```python
from build123d import *

# Parameters (mm, degrees)
CORTAR_EXTRUIR2_DEPTH = 112
CROQUIS11_W           = 4
CROQUIS11_H           = 16.808089165
CROQUIS11_W_2         = 16.808089165
CROQUIS11_H_2         = 4
CORTAR_EXTRUIR3_DEPTH = 40


with BuildPart() as part:
    # Croquis1 → Revolución1 (revolve)
    with BuildSketch(Plane.XY):
        Polygon((-27.489415048, 0), (-30, 0), (-30, -1), (-28.5, -1), (-27.603353842, -11), (-26.603353842, -11), (-22, -60), (0, -60), (0, -58.902540381), (-21.020029368, -58.902540381), (-25.804439037, -9.881949504), (-26.603353842, -9.881949504), align=None)
    revolve(axis=Axis((0, -60, 0), (0, 1, 0)))

    # Croquis9 → Cortar-Extruir2 (cut)
    with BuildSketch(Plane(origin=(0, 0, 0), x_dir=(1, 0, 0), z_dir=(0, 1, 0))):
        with BuildLine():
            Line((-1.75, 6.184718181), (-1.5, 19.300075922))
            ThreePointArc((-1.5, 19.300075922), (-7.408092304, 17.884716912), (-12.58655439, 14.707874734))
            Line((-12.58655439, 14.707874734), (-3.135819299, 5.610693033))
            ThreePointArc((-3.135819299, 5.610693033), (-2.459712132, 5.938270389), (-1.75, 6.184718181))
        make_face()
        with BuildLine():
            Line((3.135819299, 5.610693033), (12.58655439, 14.707874734))
            ThreePointArc((12.58655439, 14.707874734), (7.408092304, 17.884716912), (1.5, 19.300075922))
            Line((1.5, 19.300075922), (1.75, 6.184718181))
            ThreePointArc((1.75, 6.184718181), (2.459712132, 5.938270389), (3.135819299, 5.610693033))
        make_face()
        with BuildLine():
            Line((6.184718181, 1.75), (19.300075922, 1.5))
            ThreePointArc((19.300075922, 1.5), (17.884716912, 7.408092304), (14.707874734, 12.58655439))
            Line((14.707874734, 12.58655439), (5.610693033, 3.135819299))
            ThreePointArc((5.610693033, 3.135819299), (5.938270389, 2.459712132), (6.184718181, 1.75))
        make_face()
        with BuildLine():
            Line((5.610693033, -3.135819299), (14.707874734, -12.58655439))
            ThreePointArc((14.707874734, -12.58655439), (17.884716912, -7.408092304), (19.300075922, -1.5))
            Line((19.300075922, -1.5), (6.184718181, -1.75))
            ThreePointArc((6.184718181, -1.75), (5.938270389, -2.459712132), (5.610693033, -3.135819299))
        make_face()
        with BuildLine():
            Line((1.75, -6.184718181), (1.5, -19.300075922))
            ThreePointArc((1.5, -19.300075922), (7.408092304, -17.884716912), (12.58655439, -14.707874734))
            Line((12.58655439, -14.707874734), (3.135819299, -5.610693033))
            ThreePointArc((3.135819299, -5.610693033), (2.459712132, -5.938270389), (1.75, -6.184718181))
        make_face()
        with BuildLine():
            Line((-3.135819299, -5.610693033), (-12.58655439, -14.707874734))
            ThreePointArc((-12.58655439, -14.707874734), (-7.408092304, -17.884716912), (-1.5, -19.300075922))
            Line((-1.5, -19.300075922), (-1.75, -6.184718181))
            ThreePointArc((-1.75, -6.184718181), (-2.459712132, -5.938270389), (-3.135819299, -5.610693033))
        make_face()
        with BuildLine():
            Line((-6.184718181, -1.75), (-19.300075922, -1.5))
            ThreePointArc((-19.300075922, -1.5), (-17.884716912, -7.408092304), (-14.707874734, -12.58655439))
            Line((-14.707874734, -12.58655439), (-5.610693033, -3.135819299))
            ThreePointArc((-5.610693033, -3.135819299), (-5.938270389, -2.459712132), (-6.184718181, -1.75))
        make_face()
        with BuildLine():
            Line((-5.610693033, 3.135819299), (-14.707874734, 12.58655439))
            ThreePointArc((-14.707874734, 12.58655439), (-17.884716912, 7.408092304), (-19.300075922, 1.5))
            Line((-19.300075922, 1.5), (-6.184718181, 1.75))
            ThreePointArc((-6.184718181, 1.75), (-5.938270389, 2.459712132), (-5.610693033, 3.135819299))
        make_face()
    extrude(amount=-CORTAR_EXTRUIR2_DEPTH, mode=Mode.SUBTRACT)

    # Croquis11 → Cortar-Extruir3 (cut)
    with BuildSketch(Plane(origin=(0, -56, 0), x_dir=(1, 0, 0), z_dir=(0, 1, 0))):
        with Locations((-0.4, 22.457977408)):
            Rectangle(CROQUIS11_W, CROQUIS11_H)
        Polygon((9.372703114, 29.283983817), (2.940525861, 13.755334257), (6.636043991, 12.224600528), (13.068221244, 27.753250088), align=None)
        Polygon((19.645373498, 23.320848212), (7.760259671, 11.435734384), (10.588686796, 8.60730726), (22.473800623, 20.492421087), align=None)
        Polygon((26.854090209, 13.880448514), (11.325440649, 7.448271261), (12.856174379, 3.75275313), (28.384823939, 10.184930384), align=None)
        with Locations((21.497346893, 0.4)):
            Rectangle(CROQUIS11_W_2, CROQUIS11_H_2)
        Polygon((28.323353302, -9.372703114), (12.794703741, -2.940525861), (11.263970012, -6.636043991), (26.792619572, -13.068221244), align=None)
        Polygon((22.360217696, -19.645373498), (10.475103869, -7.760259671), (7.646676744, -10.588686796), (19.531790571, -22.473800623), align=None)
        Polygon((12.919817998, -26.854090209), (6.487640745, -11.325440649), (2.792122615, -12.856174379), (9.224299868, -28.384823939), align=None)
        with Locations((-0.560630516, -21.497346893)):
            Rectangle(CROQUIS11_W, CROQUIS11_H)
        Polygon((-10.333333629, -28.323353302), (-3.901156376, -12.794703741), (-7.596674506, -11.263970012), (-14.028851759, -26.792619572), align=None)
        Polygon((-20.606004014, -22.360217696), (-8.720890187, -10.475103869), (-11.549317311, -7.646676744), (-23.434431139, -19.531790571), align=None)
        Polygon((-27.814720725, -12.919817998), (-12.286071165, -6.487640745), (-13.816804894, -2.792122615), (-29.345454454, -9.224299868), align=None)
        with Locations((-22.457977408, 0.560630516)):
            Rectangle(CROQUIS11_W_2, CROQUIS11_H_2)
        Polygon((-29.283983817, 10.333333629), (-13.755334257, 3.901156376), (-12.224600528, 7.596674506), (-27.753250088, 14.028851759), align=None)
        Polygon((-23.320848212, 20.606004014), (-11.435734384, 8.720890187), (-8.60730726, 11.549317311), (-20.492421087, 23.434431139), align=None)
        Polygon((-13.880448514, 27.814720725), (-7.448271261, 12.286071165), (-3.75275313, 13.816804894), (-10.184930384, 29.345454454), align=None)
    extrude(amount=CORTAR_EXTRUIR3_DEPTH, mode=Mode.SUBTRACT)


solid = part.part
```
Geometry check sheet. Reference: the model listing, model coordinates, mm. A direction names the side the tool comes from. Round coordinates to 2 decimals unless told otherwise and drop trailing zeros. Loops run counter-clockwise (first coordinate to the right, second up) from the corner with the lowest first, then second, coordinate; pieces in that order, holes last. Notation, with made-up numbers: M -16,56 L 9,56 A34 ccw 9,86 Z; hole C 65,-26.75 d8. An arc over 180 degrees is marked long. Return JSON: item names as keys, results as strings. Group by question number.
(1) Set-up check for faces 5 (the face through (15.3, -56, 15.4)), 6 (the face through (-7.927, -59.444, -10.223)): record each of +Z, -Z, +X, -X, +Y, -Y from which the full face is reachable in a straight line by a thin tool's end or side.
(2) Go/stop test with flat-tipped pins: pin 1 (1 mm diameter, centred on x = 17, z = 19, fed in from -Y); pin 2 (1.5 mm diameter, centred on x = 24, y = -31, fed in from -Z); pin 3 (0.6 mm diameter, centred on x = 21.5, z = -1, fed in from +Y). Record where each tip stops, or that it passes through.
(3) Section check D-D, the plane y = -7.5. Enter the section's corners in (x, z), and give its area (3 significant figures).
(4) Section check C-C, the plane y = -42. Give the number of separate pieces and of enclosed holes in the cut face, and give its area (3 significant figures).
(5) Section check B-B, the plane x = 0. Enter the section's corners in (y, z), and give its area (3 significant figures).
(6) Mould release check, pull along Z, two halves, no side actions. Record for faces 1 (the face through (23.4, -16, -10.3)), 2 (the face through (-18.081, -36.093, -15.366)), 3 (the face through (1.6, -36, -24)), 4 (the face through (7.329, -59.444, 17.917)): pulls with the +Z half, pulls with the -Z half, needs draft (parallel to the pull), parting line crosses it, or undercut.
(7) Scan lines: line 1 along Y through (x, z) = (14.5, -1); line 2 along X through (y, z) = (-13, -1); line 3 along Y through (x, z) = (26, -2). Record each from-to range of solid material in increasing order. Write a range as [from, to].
(8) Section check A-A, the plane z = 0. Enter the section's corners in (x, y), and give its area (3 significant figures).
Data:
{
 "1": {"face 5": "+Y", "face 6": "+Y, -Y"},
 "2": {"pin 1": "y = -16", "pin 2": "z = -8.12", "pin 3": "y = -56"},
 "3": {"outline": "C 0,0 d55.83; hole C 0,0 d53.63", "area": "189 mm²"},
 "4": {"separate pieces": "16", "enclosed holes": "0", "area": "83.3 mm²"},
 "5": {"outline": "M -60,-22 L -56,-22.38 L -56,-21.3 L -58.9,-21.02 L -58.9,21.02 L -56,21.3 L -56,22.38 L -60,22 Z; M -16,-26.13 L -11,-26.6 L -11,-27.6 L -1,-28.5 L -1,-30 L 0,-30 L 0,-27.49 L -9.88,-26.6 L -9.88,-25.8 L -16,-25.21 Z; M -16,25.21 L -9.88,25.8 L -9.88,26.6 L 0,27.49 L 0,30 L -1,30 L -1,28.5 L -11,27.6 L -11,26.6 L -16,26.13 Z", "area": "92.7 mm²"},
 "6": {"face 1": "undercut", "face 2": "pulls with the -Z half", "face 3": "needs draft", "face 4": "undercut"},
 "7": {"line 1": "[-60, -58.9]", "line 2": "[-26.4, -25.48], [25.48, 26.4]", "line 3": "[-16, -9.88]"},
 "8": {"outline": "M -30,-1 L -28.5,-1 L -27.6,-11 L -26.6,-11 L -26.13,-16 L -25.21,-16 L -25.8,-9.88 L -26.6,-9.88 L -27.49,0 L -30,0 Z; M -22.38,-56 L -22,-60 L 22,-60 L 22.38,-56 L 21.3,-56 L 21.02,-58.9 L -21.02,-58.9 L -21.3,-56 Z; M 25.21,-16 L 26.13,-16 L 26.6,-11 L 27.6,-11 L 28.5,-1 L 30,-1 L 30,0 L 27.49,0 L 26.6,-9.88 L 25.8,-9.88 Z", "area": "92.7 mm²"}
}
